Check sheet for the modelled part. Datum: model origin and axes. Units: mm. A direction names the side the tool comes from. Give positions to 0.01 mm unless a question says otherwise; leave off trailing zeros. Write each loop counter-clockwise with the first axis right and the second up, starting at its lowest first coordinate (ties: lowest second). Pieces come first, ordered by that corner, then holes.
from build123d import *

# Parameters (mm, degrees)
SKETCH1_W               = 41.9
SKETCH1_H               = 41.9
BOSS_EXTRUDE1_DEPTH     = 34.3
SKETCH2_R               = 11
BOSS_EXTRUDE2_DEPTH     = 2.5
SKETCH3_R               = 2.5
BOSS_EXTRUDE3_DEPTH     = 14
SKETCH4_R               = 1.25
CUT_EXTRUDE1_DEPTH      = 7.9
MIRROR2_COPY_1_SKETCH_R = 1.25
MIRROR2_COPY_1_DEPTH    = 7.9
CUT_EXTRUDE2_DEPTH      = 15.7
MIRROR4_COPY_1_DEPTH    = 15.7
BOSS_EXTRUDE4_DEPTH     = 10.3
SKETCH12_R              = 4
CUT_EXTRUDE3_DEPTH      = 3


with BuildPart() as part:
    # Sketch1 → Boss-Extrude1 (new body)
    with BuildSketch(Plane(origin=(0, 0, 0), x_dir=(1, 0, 0), z_dir=(0, 1, 0))):
        Rectangle(SKETCH1_W, SKETCH1_H)
    extrude(amount=BOSS_EXTRUDE1_DEPTH)

    # Sketch2 → Boss-Extrude2 (add)
    with BuildSketch(Plane(origin=(0, 34.3, 0), x_dir=(1, 0, 0), z_dir=(0, 1, 0))):
        Circle(SKETCH2_R)
    extrude(amount=BOSS_EXTRUDE2_DEPTH)

    # Sketch3 → Boss-Extrude3 (add)
    with BuildSketch(Plane(origin=(0, 36.8, 0), x_dir=(1, 0, 0), z_dir=(0, 1, 0))):
        Circle(SKETCH3_R)
    extrude(amount=BOSS_EXTRUDE3_DEPTH)

    # Sketch4 → Cut-Extrude1 (cut)
    with BuildSketch(Plane(origin=(0, 34.3, 0), x_dir=(1, 0, 0), z_dir=(0, 1, 0))):
        with Locations((15.55, 15.55)):
            Circle(SKETCH4_R)
    cut_extrude1 = extrude(amount=-CUT_EXTRUDE1_DEPTH, mode=Mode.SUBTRACT)

    # Mirror1: Cut-Extrude1 across plane
    add(cut_extrude1.mirror(Plane(origin=(0, 0, 0), x_dir=(0, 0, 1), z_dir=(1, 0, 0))), mode=Mode.SUBTRACT)

    # Mirror2: Cut-Extrude1 across plane
    add(cut_extrude1.mirror(Plane.XY), mode=Mode.SUBTRACT)

    # Mirror2 copy 1 sketch → Mirror2 copy 1 (cut)
    with BuildSketch(Plane(origin=(0, 34.3, 0), x_dir=(-1, 0, 0), z_dir=(0, 1, 0))):
        with Locations((15.55, 15.55)):
            Circle(MIRROR2_COPY_1_SKETCH_R)
    extrude(amount=-MIRROR2_COPY_1_DEPTH, mode=Mode.SUBTRACT)

    # Sketch10 → Cut-Extrude2 (cut)
    with BuildSketch(Plane(origin=(0, 25.8, 0), x_dir=(-1, 0, 0), z_dir=(0, -1, 0))):
        Polygon((-20.95, 13.9), (-13.9, 20.95), (-20.95, 20.95), align=None)
    cut_extrude2 = extrude(amount=CUT_EXTRUDE2_DEPTH, mode=Mode.SUBTRACT)

    # Mirror3: Cut-Extrude2 across plane
    add(cut_extrude2.mirror(Plane(origin=(0, 0, 0), x_dir=(0, 0, 1), z_dir=(1, 0, 0))), mode=Mode.SUBTRACT)

    # Mirror4: Cut-Extrude2 across plane
    add(cut_extrude2.mirror(Plane.XY), mode=Mode.SUBTRACT)

    # Mirror4 copy 1 sketch → Mirror4 copy 1 (cut)
    with BuildSketch(Plane.XZ.offset(-25.8)):
        Polygon((-20.95, 13.9), (-13.9, 20.95), (-20.95, 20.95), align=None)
    extrude(amount=MIRROR4_COPY_1_DEPTH, mode=Mode.SUBTRACT)

    # Sketch11 → Boss-Extrude4 (add)
    with BuildSketch(Plane.XZ):
        Polygon((0, 20.95), (9.4, 20.95), (9.4, 26.95), (-9.4, 26.95), (-9.4, 20.95), align=None)
    extrude(amount=-BOSS_EXTRUDE4_DEPTH)

    # Sketch12 → Cut-Extrude3 (cut)
    with BuildSketch(Plane.XZ):
        Circle(SKETCH12_R)
    extrude(amount=-CUT_EXTRUDE3_DEPTH, mode=Mode.SUBTRACT)


solid = part.part
1) Sectioned sample at D-D on z = 0. Record the boundary of the cut face in (x, y), then the cut area to 3 significant figures.
2) Sectioned sample at B-B on y = 11.5. Record the boundary of the cut face in (x, z).
3) Access from +Z, -Z, +X, -X, +Y, -Y to the whole of each face (thin tool, end or side, straight path). Record for faces 4 (the flat face through (0, 3, 0)), 5 (the flat face through (18, 10.1, 18)), 6 (the flat face through (-18, 25.8, 18)), 7 (the cylindrical face through (14.56, 30.41, 14.79)).
4) Sectioned sample at A-A on z = 15.55. Record the boundary of the cut face in (x, y).
5) Sectioned sample at C-C on x = -15.55. Record the boundary of the cut face in (y, z), then the cut area to 3 significant figures.
6) Draft check along Z on faces 1 (the cylindrical face through (-2.38, 35.53, 10.74)), 2 (the flat face through (16, 26.4, 16)), 3 (the flat face through (-18, 10.1, 18)). Enter one of: +Z half, -Z half, draft (parallel to the pull), parting line (faces both ways), or undercut.
7) Scan lines: L1, parallel to Z at x = -15.55, y = 32.5; L2, parallel to Z at x = 15, y = 30; L3, parallel to Z at x = 0, y = 1. Record each from-to range of solid material in increasing order.
8) Gauge pin test, flat ends, axial feed: pin 1 (5 mm diameter, centred on y = 7.5, z = 25, fed in from +X); pin 2 (12 mm diameter, centred on x = 15, z = -8.5, fed in from +Y); pin 3 (2 mm diameter, centred on x = 15.5, z = 15.5, fed in from +Y). Record the tip position at first contact, or that the pin passes through.
Answers below:
1. outline: (-20.95, 0) - (-4, 0) - (-4, 3) - (4, 3) - (4, 0) - (20.95, 0) - (20.95, 34.3) - (11, 34.3) - (11, 36.8) - (2.5, 36.8) - (2.5, 50.8) - (-2.5, 50.8) - (-2.5, 36.8) - (-11, 36.8) - (-11, 34.3) - (-20.95, 34.3) - close
1. area: 1,540 mm2
2. outline: (-20.95, -13.9) - (-13.9, -20.95) - (13.9, -20.95) - (20.95, -13.9) - (20.95, 13.9) - (13.9, 20.95) - (-13.9, 20.95) - (-20.95, 13.9) - close
3. face 4: -Y
3. face 5: +Z, +X
3. face 6: +Z, -X
3. face 7: +Y
4. outline: (-20.95, 0) - (20.95, 0) - (20.95, 10.1) - (19.3, 10.1) - (19.3, 25.8) - (20.95, 25.8) - (20.95, 34.3) - (16.8, 34.3) - (16.8, 26.4) - (14.3, 26.4) - (14.3, 34.3) - (-14.3, 34.3) - (-14.3, 26.4) - (-16.8, 26.4) - (-16.8, 34.3) - (-20.95, 34.3) - (-20.95, 25.8) - (-19.3, 25.8) - (-19.3, 10.1) - (-20.95, 10.1) - close
5. outline: (0, -20.95) - (10.1, -20.95) - (10.1, -19.3) - (25.8, -19.3) - (25.8, -20.95) - (34.3, -20.95) - (34.3, -16.8) - (26.4, -16.8) - (26.4, -14.3) - (34.3, -14.3) - (34.3, 14.3) - (26.4, 14.3) - (26.4, 16.8) - (34.3, 16.8) - (34.3, 20.95) - (25.8, 20.95) - (25.8, 19.3) - (10.1, 19.3) - (10.1, 20.95) - (0, 20.95) - close
5. area: 1,350 mm2
6. face 1: parting line
6. face 2: undercut
6. face 3: draft
7. L1: z = -20.95 to -16.8, -14.3 to 14.3, 16.8 to 20.95
7. L2: z = -20.95 to -16.67, -14.43 to 14.43, 16.67 to 20.95
7. L3: z = -20.95 to -4, 4 to 26.95
8. pin 1: stops at x = 9.4
8. pin 2: stops at y = 34.3
8. pin 3: stops at y = 26.4
